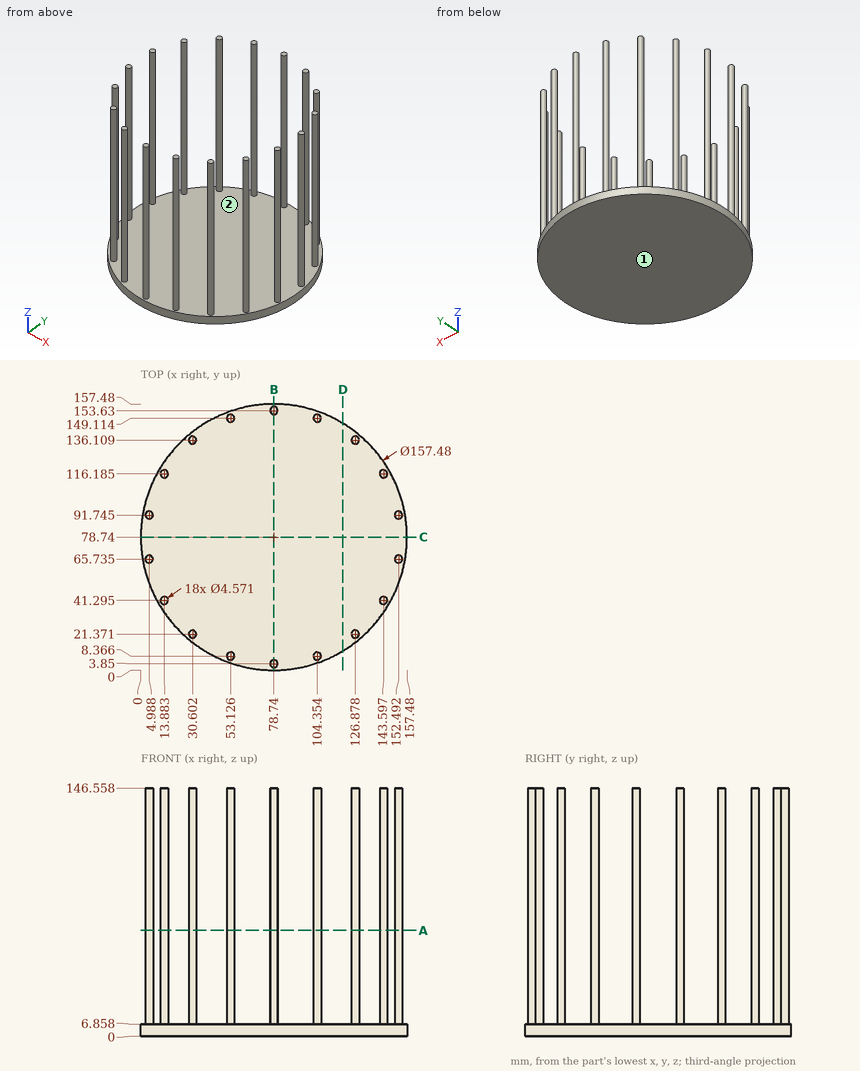
Input: dimensioned drawing with shaded views. Units: mm. Origin: part minimum x, y, z. Give positions to 0.01 mm unless a question says otherwise; leave off trailing zeros. Loops run counter-clockwise (first coordinate to the right, second up) from the corner with the lowest first, then second, coordinate; pieces in that order, holes last. Notation, with made-up numbers: M -27.75,-3.75 L -0.75,-3.75 A34 cw -0.75,33.25 Z; hole C -33.5,-23 d3. An arc over 180 degrees is marked long. Put each result on its own line as item: value.
1) First-contact query: P1, Ø12, axis at x = 67, y = 131, coming from the +Z side; P2, Ø4, axis at y = 114, z = 77.5, coming from the +X side (1 decimal); P3, Ø6, axis at x = 141.5, z = 120, coming from the +Y side; P4, Ø12, axis at x = 41, y = 114.5, coming from the -Z side. Flat tips, straight axial feed; report the tip coordinate or a pass-through.
Computed values:
P1: stops at z = 6.86
P2: stops at x = 145.9
P3: stops at y = 118.47
P4: stops at z = 0
2) Cut plane C-C, the plane y = 78.74. Return the cut outline in (x, z), plus the area to 3 significant figures.
Computed values:
outline: M 0,0 L 157.48,0 L 157.48,6.86 L 0,6.86 Z
area: 1,080 mm^2
3) Cut plane A-A, the plane z = 62.5. Give the number of separate pieces and of enclosed holes in the cut face.
Computed values:
separate pieces: 18
enclosed holes: 0
4) Material intervals for L1, parallel to Y at x = 30.5, z = 52 (1 decimal); L2, parallel to X at y = 149.5, z = 71.5; L3, parallel to X at y = 137, z = 21 (1 decimal), sorted ascending. Write a range as from..to.
Computed values:
L1: y = 19.1..23.7, 133.8..138.4
L2: x = 50.87..55.38, 102.1..106.61
L3: x = 28.5..32.7, 124.8..129
5) Cut plane D-D, the plane x = 119.5. Return the cut outline in (y, z).
Computed values:
outline: M 11.37,0 L 146.11,0 L 146.11,6.86 L 11.37,6.86 Z
6) Cut plane B-B, the plane x = 78.74. Return the cut outline in (y, z) (1 decimal).
Computed values:
outline: M 0,0 L 157.5,0 L 157.5,6.9 L 155.9,6.9 L 155.9,146.6 L 151.3,146.6 L 151.3,6.9 L 6.1,6.9 L 6.1,146.6 L 1.6,146.6 L 1.6,6.9 L 0,6.9 Z
7) Mould query, pull axis Y, two halves, no side actions, for the marked faces 1 and 2. Classes: released by +Y, released by -Y, zero draft, split by the parting line, or undercut.
Computed values:
face 1: zero draft
face 2: undercut
